Geometry check sheet. Reference: drawing and pictorial views, mm from the part's lowest x, y, z. A direction names the side the tool comes from. Round coordinates to 2 decimals unless told otherwise and drop trailing zeros. Loops run counter-clockwise (first coordinate to the right, second up) from the corner with the lowest first, then second, coordinate; pieces in that order, holes last. Notation, with made-up numbers: (67, 38.25) - (109, 38.25) arc R20 cw to (109, 42.25) - close; hole circle Ø1 at (60, 80). An arc over 180 degrees is marked (long way). Answer as CSV lines item,"result". Start each with the question number.
1) Thickness scan on line 1 along Z through (x, y) = (34, 15.9); line 2 along Z through (x, y) = (9, 1.75); line 3 along Y through (x, z) = (43.5, 7). Record the ranges inside material, lowest first.
2) Depth check by flat-ended pin: P1, Ø5, axis at x = 9, z = 19.5, coming from the +Y side; P2, Ø3, axis at y = 10.5, z = 8.5, coming from the -X side; P3, Ø1.5, axis at y = 4.5, z = 11.5, coming from the +X side. Enter the tip coordinate at first touch or a pass-through.
3) Cross-section at C-C on z = 19.5. Record the boundary of the cut face in (x, y).
4) Cross-section at A-A on x = 9. Record the boundary of the cut face in (y, z), and give its area (3 significant figures).
5) Access from +Z, -Z, +X, -X, +Y, -Y to the whole of each face (thin tool, end or side, straight path). Record for the marked faces 1, 2 and 3.
6) Cross-section at B-B on z = 8. Record the boundary of the cut face in (x, y).
7) Cross-section at D-D on x = 34. Record the boundary of the cut face in (y, z), and give its area (3 significant figures).
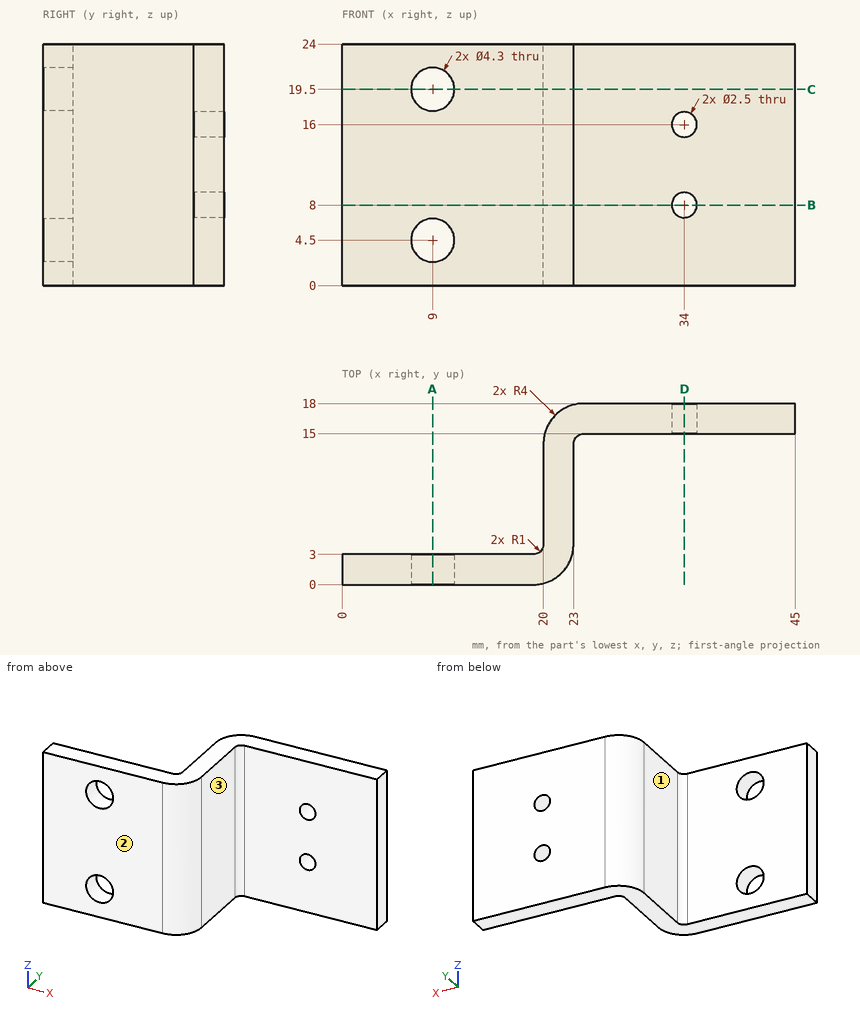
Answer block:
1,line 1,"z = 0 to 6.75, 9.25 to 14.75, 17.25 to 24"
1,line 2,"z = 0 to 2.35, 6.65 to 17.35, 21.65 to 24"
1,line 3,"y = 15 to 18"
2,P1,"stops at y = 3"
2,P2,"stops at x = 20"
2,P3,"stops at x = 23"
3,outline,"(0, 0) - (6.85, 0) - (6.85, 3) - (0, 3) - close; (11.15, 0) - (19, 0) arc R4 ccw to (23, 4) - (23, 14) arc R1 cw to (24, 15) - (45, 15) - (45, 18) - (24, 18) arc R4 ccw to (20, 14) - (20, 4) arc R1 cw to (19, 3) - (11.15, 3) - close"
4,outline,"(0, 0) - (3, 0) - (3, 2.35) - (0, 2.35) - close; (0, 6.65) - (3, 6.65) - (3, 17.35) - (0, 17.35) - close; (0, 21.65) - (3, 21.65) - (3, 24) - (0, 24) - close"
4,area,"46.2 mm^2"
5,face 1,"+Z, -Z, -X, +Y"
5,face 2,"+Z, -Z, +X, -X, -Y"
5,face 3,"+Z, -Z, +X, -Y"
6,outline,"(0, 0) - (19, 0) arc R4 ccw to (23, 4) - (23, 14) arc R1 cw to (24, 15) - (32.75, 15) - (32.75, 18) - (24, 18) arc R4 ccw to (20, 14) - (20, 4) arc R1 cw to (19, 3) - (0, 3) - close; (35.25, 15) - (45, 15) - (45, 18) - (35.25, 18) - close"
7,outline,"(15, 0) - (18, 0) - (18, 6.75) - (15, 6.75) - close; (15, 9.25) - (18, 9.25) - (18, 14.75) - (15, 14.75) - close; (15, 17.25) - (18, 17.25) - (18, 24) - (15, 24) - close"
7,area,"57.0 mm^2"
